Input: dimensioned drawing with shaded views. Units: mm. Origin: part minimum x, y, z. Give positions to 0.01 mm unless a question says otherwise; leave off trailing zeros. Loops run counter-clockwise (first coordinate to the right, second up) from the corner with the lowest first, then second, coordinate; pieces in that order, holes last. Notation, with made-up numbers: (-13, 25.25) -> (36, 25.25) arc R38 ccw to (36, 63.25) -> close; hole circle Ø3 at (-6.5, 26). An arc over 180 degrees is marked (long way). One line per question, with ' | ' between items. Start each with the question number.
Item 1: Mould query, pull axis Y, two halves, no side actions, for the marked faces 1, 2, 3 and 4. Classes: released by +Y, released by -Y, zero draft, split by the parting line, or undercut.
Item 2: Section D-D on z = 6. Return loops of the section in (x, y).
Item 3: Section C-C on y = 9. Return loops of the section in (x, z) (1 decimal), then the cut area to 3 significant figures.
Item 4: Section B-B on z = 50.5. Return loops of the section in (x, y), then the cut area to 3 significant figures.
Item 5: Pin query (flat end, axial travel): P1, Ø0.9, axis at y = 18.5, z = 45.5, coming from the -X side; P2, Ø3, axis at x = 11, z = 14, coming from the -Y side; P3, Ø0.9, axis at y = 19, z = 38.5, coming from the +X side (1 decimal). Return the tip coordinate at first contact, or that it passes through.
Item 6: Material intervals for line 1 along Y through (x, z) = (12, 59); line 2 along X through (y, z) = (10.5, 36); line 3 along X through (y, z) = (18, 15.5), sorted ascending. Write a range as [from, to].
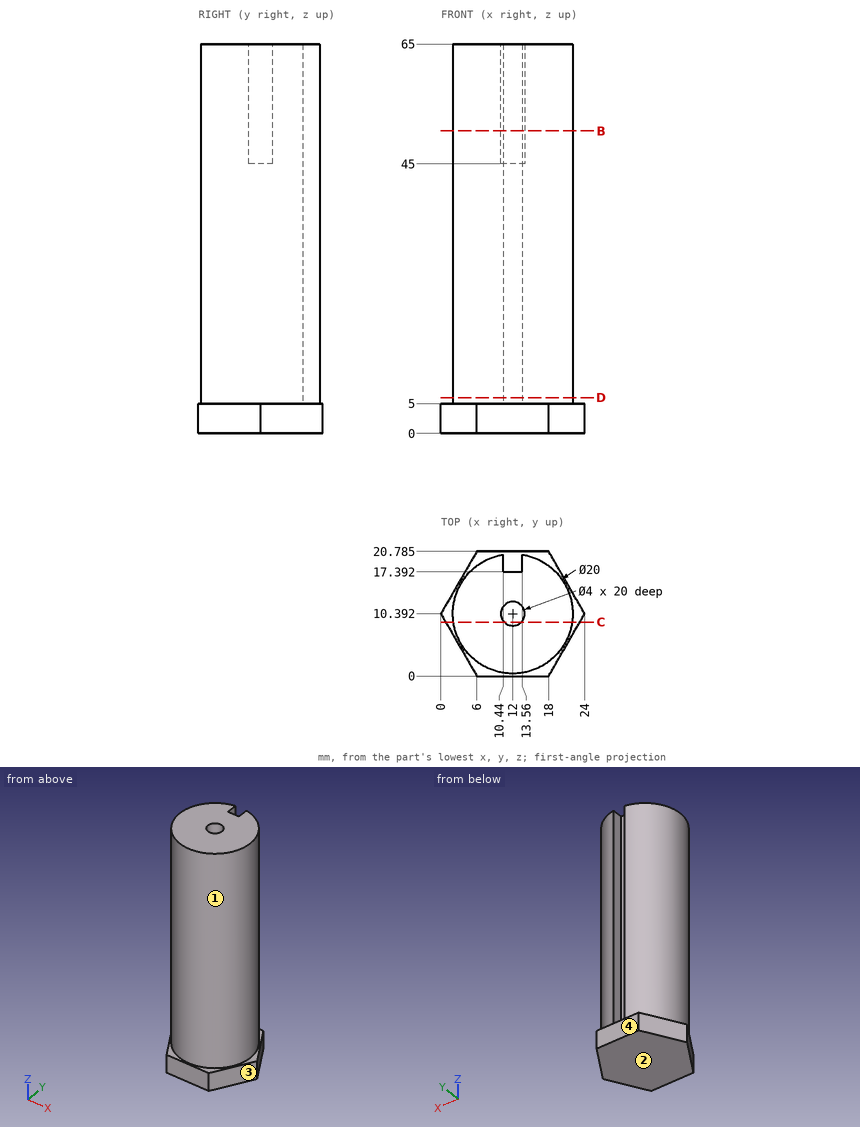
Result sheet:
1) face 1: split by the parting line | face 2: zero draft | face 3: released by -Y | face 4: released by +Y
2) outline: (10.44, 17.39) -> (10.44, 20.27) arc R10 ccw (long way) to (13.56, 20.27) -> (13.56, 17.39) -> close
3) outline: (0.8, 0) -> (23.2, 0) -> (23.2, 5) -> (21.9, 5) -> (21.9, 65) -> (13.4, 65) -> (13.4, 45) -> (10.6, 45) -> (10.6, 65) -> (2.1, 65) -> (2.1, 5) -> (0.8, 5) -> close | area: 1,240 mm²
4) outline: (10.44, 17.39) -> (10.44, 20.27) arc R10 ccw (long way) to (13.56, 20.27) -> (13.56, 17.39) -> close; hole circle Ø4 at (12, 10.39) | area: 292 mm²
5) P1: stops at x = 5.57 | P2: stops at y = 0.39 | P3: stops at x = 17.8
6) line 1: y = [0.39, 8.39], [12.39, 17.39] | line 2: x = [2, 22] | line 3: x = [5.51, 10.44], [13.56, 18.49]
